```python
from build123d import *

# Parameters (mm, degrees)
EXTRUDE_2_DEPTH      = 3
HOLE_WIZARD_M2_5_1_D = 2.05
SKETCH_4_R           = 5.1
CUT_EXTRUDE_1_DEPTH  = 10


with BuildPart() as part:
    # 草图1 → 凸台-拉伸2 (new body)
    with BuildSketch(Plane.XY):
        with BuildLine():
            ThreePointArc((-11.779760181, 14.271379579), (-12.466737886, 13.675360013), (-13.123601243, 13.046306581))
            ThreePointArc((-13.123601243, 13.046306581), (-12.803108373, 12.120767872), (-12.365117817, 11.24469604))
            ThreePointArc((-12.365117817, 11.24469604), (-12.142820781, 10.31561124), (-12.473009262, 9.419179367))
            ThreePointArc((-12.473009262, 9.419179367), (-13.244860059, 8.856275392), (-14.199312115, 8.815830257))
            ThreePointArc((-14.199312115, 8.815830257), (-15.161802274, 8.997352368), (-16.139716175, 9.052324938))
            ThreePointArc((-16.139716175, 9.052324938), (-16.564996707, 8.248388274), (-16.950263236, 7.424527004))
            ThreePointArc((-16.950263236, 7.424527004), (-16.317069389, 6.677263239), (-15.592181711, 6.018571022))
            ThreePointArc((-15.592181711, 6.018571022), (-15.049271757, 5.2325282), (-15.033334803, 4.277352535))
            ThreePointArc((-15.033334803, 4.277352535), (-15.549719866, 3.473635543), (-16.425109435, 3.091133726))
            ThreePointArc((-16.425109435, 3.091133726), (-17.388178129, 2.912706505), (-18.319914067, 2.610703653))
            ThreePointArc((-18.319914067, 2.610703653), (-18.426060932, 1.707425992), (-18.487698254, 0.800023914))
            ThreePointArc((-18.487698254, 0.800023914), (-17.627319769, 0.331957205), (-16.713435066, -0.020395362))
            ThreePointArc((-16.713435066, -0.020395362), (-15.923235192, -0.557236769), (-15.563325175, -1.442154458))
            ThreePointArc((-15.563325175, -1.442154458), (-15.754503841, -2.378138035), (-16.432604711, -3.051037542))
            ThreePointArc((-16.432604711, -3.051037542), (-17.266184176, -3.565316511), (-18.02590605, -4.183507626))
            ThreePointArc((-18.02590605, -4.183507626), (-17.798583527, -5.064133631), (-17.528267179, -5.932526839))
            ThreePointArc((-17.528267179, -5.932526839), (-16.556902937, -6.058181489), (-15.577446402, -6.056607239))
            ThreePointArc((-15.577446402, -6.056607239), (-14.64667748, -6.271743824), (-13.991402244, -6.966890501))
            ThreePointArc((-13.991402244, -6.966890501), (-13.831554774, -7.908730892), (-14.220785664, -8.781149285))
            ThreePointArc((-14.220785664, -8.781149285), (-14.812296375, -9.561823776), (-15.297399536, -10.412713019))
            ThreePointArc((-15.297399536, -10.412713019), (-14.767308791, -11.151753946), (-14.201546494, -11.863856968))
            ThreePointArc((-14.201546494, -11.863856968), (-13.250384619, -11.630129203), (-12.337637284, -11.274840748))
            ThreePointArc((-12.337637284, -11.274840748), (-11.392004814, -11.139217123), (-10.52986291, -11.550709376))
            ThreePointArc((-10.52986291, -11.550709376), (-10.040577591, -12.371205819), (-10.088370713, -13.325318158))
            ThreePointArc((-10.088370713, -13.325318158), (-10.357925871, -14.266953756), (-10.502894449, -15.23562382))
            ThreePointArc((-10.502894449, -15.23562382), (-9.741627174, -15.733268097), (-8.956828262, -16.192907475))
            ThreePointArc((-8.956828262, -16.192907475), (-8.154328435, -15.631363523), (-7.431561886, -14.970344538))
            ThreePointArc((-7.431561886, -14.970344538), (-6.598778773, -14.502277424), (-5.646207243, -14.574540946))
            ThreePointArc((-5.646207243, -14.574540946), (-4.893564768, -15.162880849), (-4.593465396, -16.069828976))
            ThreePointArc((-4.593465396, -16.069828976), (-4.504660083, -17.045252575), (-4.289915268, -18.000879201))
            ThreePointArc((-4.289915268, -18.000879201), (-3.400284827, -18.18991721), (-2.502440741, -18.335016099))
            ThreePointArc((-2.502440741, -18.335016099), (-1.956985011, -17.521495584), (-1.521812876, -16.644020345))
            ThreePointArc((-1.521812876, -16.644020345), (-0.914351093, -15.9067248), (0, -15.63))
            ThreePointArc((0, -15.63), (0.914351093, -15.9067248), (1.521812876, -16.644020345))
            ThreePointArc((1.521812876, -16.644020345), (1.956985011, -17.521495584), (2.502440741, -18.335016099))
            ThreePointArc((2.502440741, -18.335016099), (3.400284827, -18.18991721), (4.289915268, -18.000879201))
            ThreePointArc((4.289915268, -18.000879201), (4.504660083, -17.045252575), (4.593465396, -16.069828976))
            ThreePointArc((4.593465396, -16.069828976), (4.893564768, -15.162880849), (5.646207243, -14.574540946))
            ThreePointArc((5.646207243, -14.574540946), (6.598778773, -14.502277424), (7.431561886, -14.970344538))
            ThreePointArc((7.431561886, -14.970344538), (8.154328435, -15.631363523), (8.956828262, -16.192907475))
            ThreePointArc((8.956828262, -16.192907475), (9.741627174, -15.733268097), (10.502894449, -15.23562382))
            ThreePointArc((10.502894449, -15.23562382), (10.357925871, -14.266953756), (10.088370713, -13.325318158))
            ThreePointArc((10.088370713, -13.325318158), (10.040577591, -12.371205819), (10.52986291, -11.550709376))
            ThreePointArc((10.52986291, -11.550709376), (11.392004814, -11.139217123), (12.337637284, -11.274840748))
            ThreePointArc((12.337637284, -11.274840748), (13.250384619, -11.630129203), (14.201546494, -11.863856968))
            ThreePointArc((14.201546494, -11.863856968), (14.767308791, -11.151753946), (15.297399536, -10.412713019))
            ThreePointArc((15.297399536, -10.412713019), (14.812296375, -9.561823776), (14.220785664, -8.781149285))
            ThreePointArc((14.220785664, -8.781149285), (13.831554774, -7.908730892), (13.991402244, -6.966890501))
            ThreePointArc((13.991402244, -6.966890501), (14.64667748, -6.271743824), (15.577446402, -6.056607239))
            ThreePointArc((15.577446402, -6.056607239), (16.556902937, -6.058181489), (17.528267179, -5.932526839))
            ThreePointArc((17.528267179, -5.932526839), (17.798583527, -5.064133631), (18.02590605, -4.183507626))
            ThreePointArc((18.02590605, -4.183507626), (17.266184176, -3.565316511), (16.432604711, -3.051037542))
            ThreePointArc((16.432604711, -3.051037542), (15.754503841, -2.378138035), (15.563325175, -1.442154458))
            ThreePointArc((15.563325175, -1.442154458), (15.923235192, -0.557236769), (16.713435066, -0.020395362))
            ThreePointArc((16.713435066, -0.020395362), (17.627319769, 0.331957205), (18.487698254, 0.800023914))
            ThreePointArc((18.487698254, 0.800023914), (18.426060932, 1.707425992), (18.319914067, 2.610703653))
            ThreePointArc((18.319914067, 2.610703653), (17.388178129, 2.912706505), (16.425109435, 3.091133726))
            ThreePointArc((16.425109435, 3.091133726), (15.549719866, 3.473635543), (15.033334803, 4.277352535))
            ThreePointArc((15.033334803, 4.277352535), (15.049271757, 5.2325282), (15.592181711, 6.018571022))
            ThreePointArc((15.592181711, 6.018571022), (16.317069389, 6.677263239), (16.950263236, 7.424527004))
            ThreePointArc((16.950263236, 7.424527004), (16.564996707, 8.248388274), (16.139716175, 9.052324938))
            ThreePointArc((16.139716175, 9.052324938), (15.161802274, 8.997352368), (14.199312115, 8.815830257))
            ThreePointArc((14.199312115, 8.815830257), (13.244860059, 8.856275392), (12.473009262, 9.419179367))
            ThreePointArc((12.473009262, 9.419179367), (12.142820781, 10.31561124), (12.365117817, 11.24469604))
            ThreePointArc((12.365117817, 11.24469604), (12.803108373, 12.120767872), (13.123601243, 13.046306581))
            ThreePointArc((13.123601243, 13.046306581), (12.466737886, 13.675360013), (11.779760181, 14.271379579))
            ThreePointArc((11.779760181, 14.271379579), (10.887741008, 13.866855937), (10.055819013, 13.349900061))
            ThreePointArc((10.055819013, 13.349900061), (9.151208508, 13.042826175), (8.228134706, 13.288893831))
            ThreePointArc((8.228134706, 13.288893831), (7.596414573, 14.005513822), (7.468076245, 14.952162548))
            ThreePointArc((7.468076245, 14.952162548), (7.560016626, 15.927295641), (7.524524182, 16.906110163))
            ThreePointArc((7.524524182, 16.906110163), (6.684777033, 17.255398605), (5.8288823, 17.563005328))
            ThreePointArc((5.8288823, 17.563005328), (5.143229987, 16.863563773), (4.554231832, 16.080991887))
            ThreePointArc((4.554231832, 16.080991887), (3.821635541, 15.46787101), (2.872004963, 15.363869548))
            ThreePointArc((2.872004963, 15.363869548), (2.024070484, 15.803894155), (1.562429593, 16.640256651))
            ThreePointArc((1.562429593, 16.640256651), (1.295902743, 17.582753877), (0.909218435, 18.482649887))
            ThreePointArc((0.909218435, 18.482649887), (0, 18.505), (-0.909218435, 18.482649887))
            ThreePointArc((-0.909218435, 18.482649887), (-1.295902743, 17.582753877), (-1.562429593, 16.640256651))
            ThreePointArc((-1.562429593, 16.640256651), (-2.024070484, 15.803894155), (-2.872004963, 15.363869548))
            ThreePointArc((-2.872004963, 15.363869548), (-3.821635541, 15.46787101), (-4.554231832, 16.080991887))
            ThreePointArc((-4.554231832, 16.080991887), (-5.143229987, 16.863563773), (-5.8288823, 17.563005328))
            ThreePointArc((-5.8288823, 17.563005328), (-6.684777033, 17.255398605), (-7.524524182, 16.906110163))
            ThreePointArc((-7.524524182, 16.906110163), (-7.560016626, 15.927295641), (-7.468076245, 14.952162548))
            ThreePointArc((-7.468076245, 14.952162548), (-7.596414573, 14.005513822), (-8.228134706, 13.288893831))
            ThreePointArc((-8.228134706, 13.288893831), (-9.151208508, 13.042826175), (-10.055819013, 13.349900061))
            ThreePointArc((-10.055819013, 13.349900061), (-10.887741008, 13.866855937), (-11.779760181, 14.271379579))
        make_face()
    extrude(amount=EXTRUDE_2_DEPTH)

    # M2.5 螺纹孔1 (through all)
    with Locations(Plane(origin=(0, 7.2, 3), x_dir=(1, 0, 0), z_dir=(0, 0, 1))):
        with Locations((0, 0), (7.2, -7.2), (0, -14.4), (-7.2, -7.2)):
            Hole(HOLE_WIZARD_M2_5_1_D / 2)

    # 草图4 → 切除-拉伸1 (cut)
    with BuildSketch(Plane(origin=(0, 0, 0), x_dir=(-1, 0, 0), z_dir=(0, 0, -1))):
        Circle(SKETCH_4_R)
    extrude(amount=-CUT_EXTRUDE_1_DEPTH, mode=Mode.SUBTRACT)


solid = part.part
```
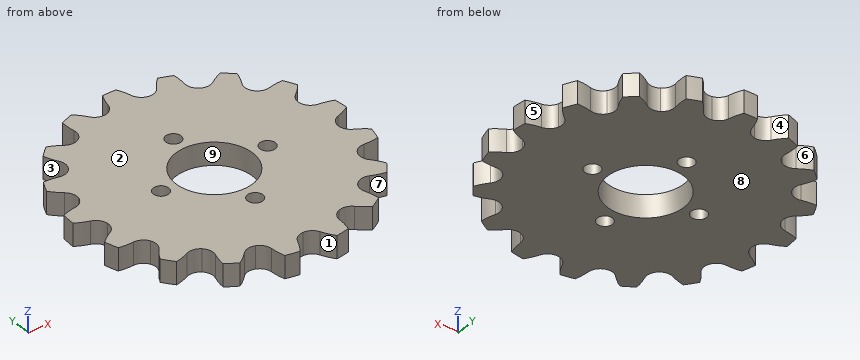
Read the model definition and answer for the solid it produces. Units are mm, in the model's axes. Face numbers are marked on the shaded views. A direction names the side the tool comes from. Give positions to 0.01 mm unless a question says otherwise; leave off trailing zeros.
(1) For the marked faces 1, 2, 3, 4 and 5, determine the directions among +Z, -Z, +X, -X, +Y, -Y from which every point of the face is accessible in a straight line to the end or side of a thin tool.
(2) Find section A-A (z = 2). Give the number of separate pieces and of enclosed holes in the cut face, plus the area to 3 significant figures.
(3) For a pull along Y with two mould halves and no side action, classify the marked faces 6, 7, 8 and 9 as released by +Y, released by -Y, zero draft, split by the parting line, or undercut.
(4) Given pin 1 (1.8 mm diameter, centred on x = -7.2, y = 0, fed in from +Z); pin 2 (3 mm diameter, centred on x = 7.5, y = 8, fed in from -Z); pin 3 (1.5 mm diameter, centred on x = 5, z = 1.5, fed in from +Y), each flat-ended and moving along its own axis, determine where each tip first touches the part or whether it passes through.
(5) Straight lines are drawn through the part: L1, parallel to Y at x = 17.5, z = 0.75; L2, parallel to Y at x = -8, z = 0.1; L3, parallel to X at y = 12.5, z = 2.4. For each, find the intervals that lie inside material, in ascending order.
Result sheet:
1. face 1: +Z, -Z, -Y
1. face 2: +Z, +X, -X, +Y, -Y
1. face 3: +Z, -Z, -X
1. face 4: +Z, -Z, +Y
1. face 5: +Z, -Z, +X
2. separate pieces: 1
2. enclosed holes: 5
2. area: 820 mm2
3. face 6: released by +Y
3. face 7: released by -Y
3. face 8: zero draft
3. face 9: undercut
4. pin 1: passes through
4. pin 2: stops at z = 0
4. pin 3: stops at y = 17.49
5. L1: y = -5.94 to -3.74, 0.27 to 2.88
5. L2: y = -15.5 to -0.64, 0.64 to 13.46
5. L3: x = -12.95 to 12.95
